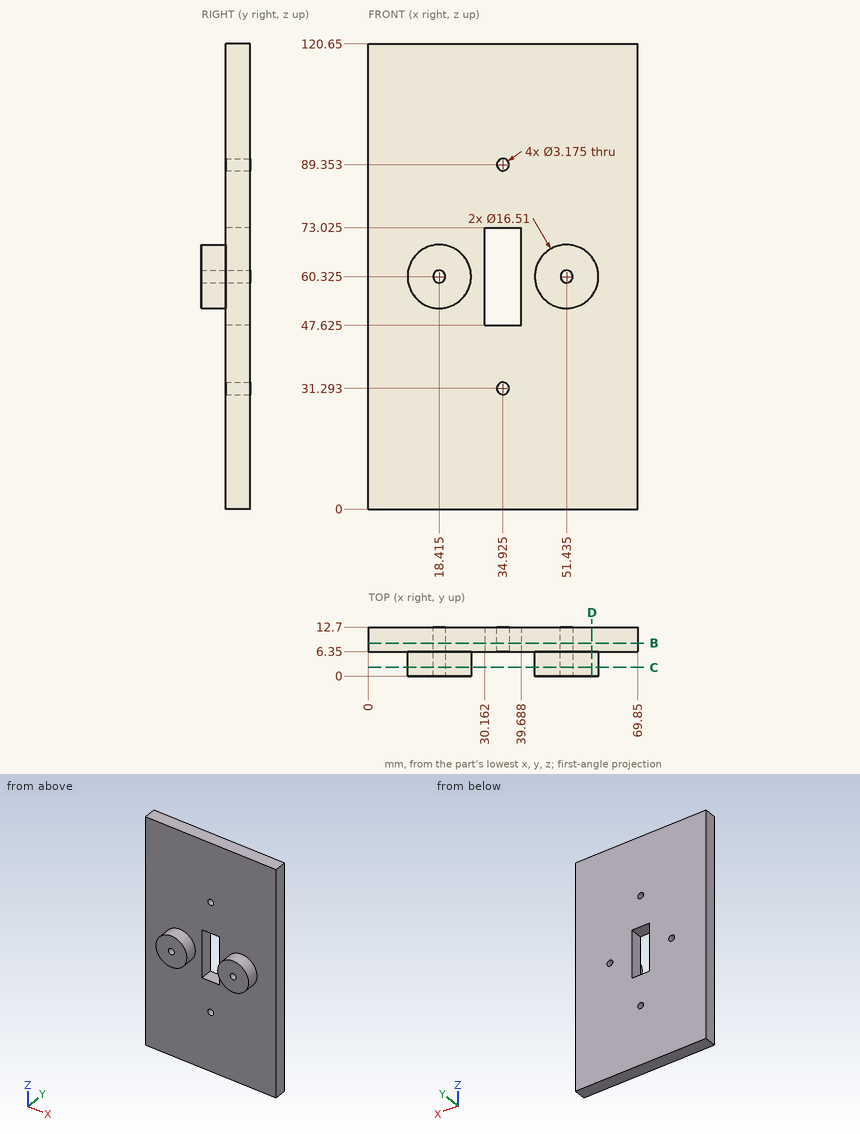
Job drawing, mm, ordinate dimensions from the low corner. One solid piece. Round coordinates to 2 decimals unless told otherwise and drop trailing zeros. Loops run counter-clockwise (first coordinate to the right, second up) from the corner with the lowest first, then second, coordinate; pieces in that order, holes last. Notation, with made-up numbers: (64, -37.5) -> (104, -37.5) arc R23 cw to (104, -9.5) -> close; hole circle Ø8 at (-24.75, -21). An arc over 180 degrees is marked (long way). Use CSV: the item, a comma, the result in double quotes. Start each with the question number.
Q1. Drill centre lines: L1, parallel to Y at x = 31, z = 43.5; L2, parallel to X at y = 0.5, z = 59 (1 decimal); L3, parallel to X at y = 6, z = 57.5. Where is each one in solid material? Low to high.
Q2. Flat gauge pins, fed straight in: pin 1 Ø6 at (x, z) = (21, 32) entering from -Y; pin 2 Ø6 at (y, z) = (1.5, 59) entering from +X. Where does each tip first touch, or does it go through?
Q3. Saw through at C-C on y = 2.25. Give the cut face in (x, z) (1 decimal), and give its area (3 significant figures).
Q4. Saw through at B-B on y = 8.5. Count the separate pieces of the cut face and the enclosed holes in it, and give its area (3 significant figures).
Q5. Saw through at D-D on x = 58. Give the cut face in (y, z).
Solutions:
1,L1,"y = 6.35 to 12.7"
1,L2,"x = 10.3 to 17.5, 19.3 to 26.6, 43.3 to 50.6, 52.3 to 59.6"
1,L3,"x = 10.66 to 26.17, 43.68 to 59.19"
2,pin 1,"stops at y = 6.35"
2,pin 2,"stops at x = 59.69"
3,outline,"circle Ø16.5 at (18.4, 60.3); circle Ø16.5 at (51.4, 60.3); hole circle Ø3.2 at (18.4, 60.3); hole circle Ø3.2 at (51.4, 60.3)"
3,area,"412 mm^2"
4,separate pieces,"1"
4,enclosed holes,"5"
4,area,"8,150 mm^2"
5,outline,"(0, 55.32) -> (6.35, 55.32) -> (6.35, 0) -> (12.7, 0) -> (12.7, 120.65) -> (6.35, 120.65) -> (6.35, 65.33) -> (0, 65.33) -> close"
